```python
from build123d import *

# Parameters (mm, degrees)
SKETCH3_R           = 2.921
SKETCH3_R_2         = 10
SKETCH3_R_3         = 2.75
BOSS_EXTRUDE1_DEPTH = 10
SKETCH4_W           = 10
SKETCH4_H           = 95
BOSS_EXTRUDE2_DEPTH = 70
SKETCH8_R           = 10
SKETCH8_R_2         = 2.75
CUT_EXTRUDE2_DEPTH  = 43.8
BOSS_EXTRUDE3_DEPTH = 7.5
FILLET1_R           = 5
SKETCH14_R          = 4.75
SKETCH14_R_2        = 4.445
CUT_EXTRUDE4_DEPTH  = 5.2
SKETCH15_R          = 4.75
CUT_EXTRUDE5_DEPTH  = 5.3


with BuildPart() as part:
    # Sketch3 → Boss-Extrude1 (new body)
    with BuildSketch(Plane.XY):
        with BuildLine():
            Line((163.617133813, 80.05993294), (203.617133813, 80.05993294))
            ThreePointArc((203.617133813, 80.05993294), (236.678629544, 66.053697227), (249.617133813, 32.55993294))
            ThreePointArc((249.617133813, 32.55993294), (235.791661756, -0.074873068), (203.617133813, -14.94006706))
            Line((203.617133813, -14.94006706), (163.617133813, -14.94006706))
            Line((163.617133813, -14.94006706), (68.617133813, -14.94006706))
            Line((68.617133813, -14.94006706), (68.617133813, 80.05993294))
            Line((68.617133813, 80.05993294), (163.617133813, 80.05993294))
        make_face()
        with Locations((224.617133813, 32.55993294)):
            Circle(SKETCH3_R, mode=Mode.SUBTRACT)
        with Locations((131.802603987, 32.55993294)):
            Circle(SKETCH3_R_2, mode=Mode.SUBTRACT)
        with Locations((139.802603987, 8.55993294)):
            Circle(SKETCH3_R_3, mode=Mode.SUBTRACT)
        with Locations((119.802603987, 8.55993294)):
            Circle(SKETCH3_R_3, mode=Mode.SUBTRACT)
        with Locations((105.802603987, 22.55993294)):
            Circle(SKETCH3_R_3, mode=Mode.SUBTRACT)
        with Locations((105.802603987, 42.55993294)):
            Circle(SKETCH3_R_3, mode=Mode.SUBTRACT)
        with Locations((119.802603987, 56.55993294)):
            Circle(SKETCH3_R_3, mode=Mode.SUBTRACT)
        with Locations((139.802603987, 56.55993294)):
            Circle(SKETCH3_R_3, mode=Mode.SUBTRACT)
    extrude(amount=BOSS_EXTRUDE1_DEPTH)

    # Sketch4 → Boss-Extrude2 (add)
    with BuildSketch(Plane(origin=(0, 0, 0), x_dir=(-1, 0, 0), z_dir=(0, 0, -1))):
        with Locations((-73.617133813, 32.55993294)):
            Rectangle(SKETCH4_W, SKETCH4_H)
    extrude(amount=BOSS_EXTRUDE2_DEPTH)

    # Sketch8 → Cut-Extrude2 (cut)
    with BuildSketch(Plane.ZY.offset(-68.617133813)):
        with Locations((-40, 32.55993294)):
            Circle(SKETCH8_R)
        with Locations((-56.167891819, 25.862972874)):
            Circle(SKETCH8_R_2)
        with Locations((-56.167891819, 39.256893006)):
            Circle(SKETCH8_R_2)
        with Locations((-46.696960066, 48.727824759)):
            Circle(SKETCH8_R_2)
        with Locations((-33.303039934, 48.727824759)):
            Circle(SKETCH8_R_2)
        with Locations((-23.832108181, 39.256893006)):
            Circle(SKETCH8_R_2)
        with Locations((-23.832108181, 25.862972874)):
            Circle(SKETCH8_R_2)
        with Locations((-33.303039934, 16.392041121)):
            Circle(SKETCH8_R_2)
        with Locations((-46.696960066, 16.392041121)):
            Circle(SKETCH8_R_2)
    extrude(amount=-CUT_EXTRUDE2_DEPTH, mode=Mode.SUBTRACT)

    # Sketch9 → Boss-Extrude3 (add)
    with BuildSketch(Plane.XZ.offset(14.94006706)):
        Polygon((78.617133813, -70), (153.617133813, 0), (78.617133813, 0), align=None)
    boss_extrude3 = extrude(amount=-BOSS_EXTRUDE3_DEPTH)

    # Mirror1: Boss-Extrude3 across plane
    add(boss_extrude3.mirror(Plane(origin=(0, 32.55993294, 0), x_dir=(0, 0, 1), z_dir=(0, -1, 0))))

    # Fillet1
    fillet1_edges = [part.edges().sort_by_distance(p)[0] for p in [
        (153.617133813, -11.19006706, 0),
        (153.617133813, 76.30993294, 0),
    ]]
    fillet(fillet1_edges, radius=FILLET1_R)

    # Sketch14 → Cut-Extrude4 (cut)
    with BuildSketch(Plane.XY.offset(10)):
        with Locations((119.802603987, 56.55993294)):
            Circle(SKETCH14_R)
        with Locations((139.802603987, 56.55993294)):
            Circle(SKETCH14_R)
        with Locations((105.802603987, 42.55993294)):
            Circle(SKETCH14_R)
        with Locations((119.802603987, 8.55993294)):
            Circle(SKETCH14_R)
        with Locations((139.802603987, 8.55993294)):
            Circle(SKETCH14_R)
        with Locations((105.802603987, 22.55993294)):
            Circle(SKETCH14_R)
        with Locations((224.617133813, 32.55993294)):
            Circle(SKETCH14_R_2)
    extrude(amount=-CUT_EXTRUDE4_DEPTH, mode=Mode.SUBTRACT)

    # Sketch15 → Cut-Extrude5 (cut)
    with BuildSketch(Plane(origin=(78.617133813, 0, 0), x_dir=(0, 0, -1), z_dir=(1, 0, 0))):
        with Locations((23.832108181, 39.256893006)):
            Circle(SKETCH15_R)
        with Locations((33.303039934, 48.727824759)):
            Circle(SKETCH15_R)
        with Locations((46.696960066, 48.727824759)):
            Circle(SKETCH15_R)
        with Locations((56.167891819, 39.256893006)):
            Circle(SKETCH15_R)
        with Locations((56.167891819, 25.862972874)):
            Circle(SKETCH15_R)
        with Locations((46.696960066, 16.392041121)):
            Circle(SKETCH15_R)
        with Locations((33.303039934, 16.392041121)):
            Circle(SKETCH15_R)
        with Locations((23.832108181, 25.862972874)):
            Circle(SKETCH15_R)
    extrude(amount=-CUT_EXTRUDE5_DEPTH, mode=Mode.SUBTRACT)


solid = part.part
```
The listing builds one solid part. Answer for the finished solid, in the listing's coordinates (mm). A direction names the side the tool comes from. Give positions to 0.01 mm unless a question says otherwise; leave off trailing zeros. Write each loop counter-clockwise with the first axis right and the second up, starting at its lowest first coordinate (ties: lowest second). Pieces come first, ordered by that corner, then holes. Notation, with made-up numbers: (17.25, -3) -> (37.25, -3) arc R23 cw to (37.25, 35) -> close; hole circle Ø9 at (9.25, 18.5). An arc over 180 degrees is marked (long way). Use one line per item in the form item = value.
1) Each of these flat-tipped pins is pushed along its axis until it touches: P1, Ø12.5, axis at x = 105.8, y = 22.56, coming from the -Z side; P2, Ø8, axis at y = 23, z = -53, coming from the +X side; P3, Ø7.5, axis at x = 119.5, y = 9, coming from the +Z side; P4, Ø3.5, axis at y = 39.26, z = -23.83, coming from the -X side. Where does it stop, or does it pass through?
Result:
P1 = 0
P2 = 78.62
P3 = 4.8
P4 = through
2) For a pull along Y with two mould halves and no side action, classify faces 6 (the flat face through (73.317, 45.6, -33.2)), 7 (the flat face through (114.882, -11.243, -36.153)) as +Y half, -Y half, draft (parallel to the pull), parting line (faces both ways), or undercut.
Result:
face_6 = undercut
face_7 = draft
3) Section B-B on x = 130.5 is taken. Write down the section's boundary in (y, z).
Result:
outline = (-14.94, -21.58) -> (-7.44, -21.58) -> (-7.44, 0) -> (22.65, 0) -> (22.65, 10) -> (-14.94, 10) -> close; (42.47, 0) -> (72.56, 0) -> (72.56, -21.58) -> (80.06, -21.58) -> (80.06, 10) -> (42.47, 10) -> close
4) Section A-A on z = -40 is taken. Write down the section's boundary in (x, y), plus the area to 3 significant figures.
Result:
outline = (68.62, -14.94) -> (110.76, -14.94) -> (110.76, -7.44) -> (78.62, -7.44) -> (78.62, 22.56) -> (68.62, 22.56) -> close; (68.62, 42.56) -> (78.62, 42.56) -> (78.62, 72.56) -> (110.76, 72.56) -> (110.76, 80.06) -> (68.62, 80.06) -> close
area = 1,230 mm²
5) Straight lines are drawn through the part: probe 1 along Y at (x, z) = (89, -19.5); probe 2 along X at (y, z) = (70.5, -9); probe 3 along Z at (x, y) = (171.5, 12.5). For each, find the intervals that lie inside material, in ascending order.
Result:
probe_1 = -14.94 to -7.44, 72.56 to 80.06
probe_2 = 68.62 to 78.62
probe_3 = 0 to 10
6) A tool of negligible diameter and unlimited length cuts with its end or side. For faces 1 (the cylindrical face through (73.55, 33, -49.99)), 2 (the cylindrical face through (76, 27.29, -60.7)), 3 (the cylindrical face through (137.62, 54.89, 2.37)), 4 (the cylindrical face through (220.176, 32.755, 7.436)), 5 (the flat face through (165, 33, 0)), from which of +Z, -Z, +X, -X, +Y, -Y can it reach the whole face along a straight path? Write none if from no direction.
Result:
face_1 = +X, -X
face_2 = +X
face_3 = +Z, -Z
face_4 = +Z
face_5 = -Z, +X
7) Section C-C on x = 188.5 is taken. Write down the section's boundary in (y, z), plus the area to 3 significant figures.
Result:
outline = (-14.94, 0) -> (80.06, 0) -> (80.06, 10) -> (-14.94, 10) -> close
area = 950 mm²
